from build123d import *

# Parameters (mm, degrees)
CUBE006_W                    = 20
CUBE006_H                    = 10
CUBE006_DEPTH                = 20
CUBE006_ROLL_ANGLE           = 35
CUBE006_PLACEMENT_ANGLE      = -45
CUBE008_W                    = 20
CUBE008_H                    = 10
CUBE008_DEPTH                = 20
CUBE008_ROLL_ANGLE           = 35
CUBE008_PLACEMENT_ANGLE      = -45
CUBE007_W                    = 20
CUBE007_H                    = 10
CUBE007_DEPTH                = 20
CUBE007_ROLL_ANGLE           = 35
CUBE007_PLACEMENT_ANGLE      = 45
CUBE005_W                    = 20
CUBE005_H                    = 10
CUBE005_DEPTH                = 20
CUBE005_ROLL_ANGLE           = 35
CUBE005_PLACEMENT_ANGLE      = 45
CUBE003_W                    = 4.5
CUBE003_H                    = 20
CUBE003_DEPTH                = 1.5
CUBE004_W                    = 4.5
CUBE004_H                    = 20
CUBE004_DEPTH                = 1.5
CYLINDER005_R                = 12
CYLINDER005_DEPTH            = 5
CYLINDER004_R                = 15
CYLINDER004_DEPTH            = 3.9
CUBE002_W                    = 4
CUBE002_H                    = 20
CUBE002_DEPTH                = 28.5
CYLINDER003_R                = 7.9
CYLINDER003_DEPTH            = 32.5
CUBE001_W                    = 10
CUBE001_H                    = 20
CUBE001_DEPTH                = 28.5
MATRIX_UNION_PITCH_ANGLE     = -90
MATRIX_UNION_PLACEMENT_ANGLE = 90
PRISM003_DEPTH               = 10
CYLINDER001_R                = 12
CYLINDER001_DEPTH            = 5
CYLINDER_R                   = 15
CYLINDER_DEPTH               = 3.9
DIFFERENCE_PITCH_ANGLE       = -90
DIFFERENCE_PLACEMENT_ANGLE   = 90
PRISM002_DEPTH               = 10
PRISM_DEPTH                  = 3
PRISM_PLACEMENT_ANGLE        = 30
PRISM001_DEPTH               = 3
PRISM001_PLACEMENT_ANGLE     = 30
CUBE_W                       = 26
CUBE_H                       = 14
CUBE_DEPTH                   = 3


with BuildPart() as cube006:
    # cube006 → cube006 (new body)
    with BuildSketch(Plane.XY):
        with Locations((10, 5)):
            Rectangle(CUBE006_W, CUBE006_H)
    extrude(amount=CUBE006_DEPTH)


with BuildPart() as cube006_1:
    # cube006 roll: moved
    add(cube006.part.rotate(Axis((0, 0, 0), (1, 0, 0)), CUBE006_ROLL_ANGLE))


with BuildPart() as cube006_2:
    # cube006 placement: moved
    add(cube006_1.part.moved(Location((-15.80755, -5.915414, -13.927285))).rotate(Axis((-15.80755, -5.915414, -13.927285), (0, 0, 1)), CUBE006_PLACEMENT_ANGLE))


with BuildPart() as cube008:
    # cube008 → cube008 (new body)
    with BuildSketch(Plane.XY):
        with Locations((10, 5)):
            Rectangle(CUBE008_W, CUBE008_H)
    extrude(amount=CUBE008_DEPTH)


with BuildPart() as cube008_1:
    # cube008 roll: moved
    add(cube008.part.rotate(Axis((0, 0, 0), (1, 0, 0)), CUBE008_ROLL_ANGLE))


with BuildPart() as cube008_2:
    # cube008 placement: moved
    add(cube008_1.part.moved(Location((-15.80755, -5.915414, -13.927285))).rotate(Axis((-15.80755, -5.915414, -13.927285), (0, 0, 1)), CUBE008_PLACEMENT_ANGLE))


with BuildPart() as matrix_union001:
    # cube007 → cube007 (new body)
    with BuildSketch(Plane.XY):
        with Locations((10, 5)):
            Rectangle(CUBE007_W, CUBE007_H)
    extrude(amount=CUBE007_DEPTH)


with BuildPart() as matrix_union001_1:
    # cube007 roll: moved
    add(matrix_union001.part.rotate(Axis((0, 0, 0), (1, 0, 0)), CUBE007_ROLL_ANGLE))


with BuildPart() as matrix_union001_2:
    # cube007 placement: moved
    add(matrix_union001_1.part.moved(Location((1.665414, -20.05755, -13.927285))).rotate(Axis((1.665414, -20.05755, -13.927285), (0, 0, 1)), CUBE007_PLACEMENT_ANGLE))

    # Matrix_Union001: union cube008
    add(cube008_2.part)


with BuildPart() as mirrored_matrix_union001:
    # mirr_Matrix_Union001: instance of Matrix_Union001
    add(matrix_union001_2.part.mirror(Plane(origin=(0, 0, 0), x_dir=(1, 0, 0), z_dir=(0, 1, 0))))


with BuildPart() as union005:
    # cube005 → cube005 (new body)
    with BuildSketch(Plane.XY):
        with Locations((10, 5)):
            Rectangle(CUBE005_W, CUBE005_H)
    extrude(amount=CUBE005_DEPTH)


with BuildPart() as union005_1:
    # cube005 roll: moved
    add(union005.part.rotate(Axis((0, 0, 0), (1, 0, 0)), CUBE005_ROLL_ANGLE))


with BuildPart() as union005_2:
    # cube005 placement: moved
    add(union005_1.part.moved(Location((1.665414, -20.05755, -13.927285))).rotate(Axis((1.665414, -20.05755, -13.927285), (0, 0, 1)), CUBE005_PLACEMENT_ANGLE))

    # union005: union cube006, mirrored Matrix_Union001
    add(cube006_2.part)
    add(mirrored_matrix_union001.part)


with BuildPart() as cube003:
    # cube003 → cube003 (new body)
    with BuildSketch(Plane(origin=(-10, -10, 0), x_dir=(1, 0, 0), z_dir=(0, 0, 1))):
        with Locations((2.25, 10)):
            Rectangle(CUBE003_W, CUBE003_H)
    extrude(amount=CUBE003_DEPTH)


with BuildPart() as cube004:
    # cube004 → cube004 (new body)
    with BuildSketch(Plane(origin=(-10, -10, 27), x_dir=(1, 0, 0), z_dir=(0, 0, 1))):
        with Locations((2.25, 10)):
            Rectangle(CUBE004_W, CUBE004_H)
    extrude(amount=CUBE004_DEPTH)


with BuildPart() as cylinder006:
    # cylinder006 → cylinder006 (revolve)
    with BuildSketch(Plane(origin=(0, 0, 3), x_dir=(1, 0, 0), z_dir=(0, -1, 0))):
        Polygon((0, 0), (12, 0), (15, 1), (0, 1), align=None)
    revolve(axis=Axis((0, 0, 3), (0, 0, 1)))


with BuildPart() as union004:
    # cylinder005 → cylinder005 (new body)
    with BuildSketch(Plane.XY):
        Circle(CYLINDER005_R)
    extrude(amount=CYLINDER005_DEPTH)

    # union004: union cylinder006
    add(cylinder006.part)


with BuildPart() as difference003:
    # cylinder004 → cylinder004 (new body)
    with BuildSketch(Plane.XY):
        Circle(CYLINDER004_R)
    extrude(amount=CYLINDER004_DEPTH)

    # difference003: cut union004
    add(union004.part, mode=Mode.SUBTRACT)


with BuildPart() as difference003_1:
    # difference003 placement: moved
    add(difference003.part.moved(Location((0, 0, 12.5))))


with BuildPart() as cube002:
    # cube002 → cube002 (new body)
    with BuildSketch(Plane(origin=(-14, -10, 0), x_dir=(1, 0, 0), z_dir=(0, 0, 1))):
        with Locations((2, 10)):
            Rectangle(CUBE002_W, CUBE002_H)
    extrude(amount=CUBE002_DEPTH)


with BuildPart() as cylinder003:
    # cylinder003 → cylinder003 (new body)
    with BuildSketch(Plane.XY.offset(-2)):
        Circle(CYLINDER003_R)
    extrude(amount=CYLINDER003_DEPTH)


with BuildPart() as difference005:
    # cube001 → cube001 (new body)
    with BuildSketch(Plane(origin=(-10, -10, 0), x_dir=(1, 0, 0), z_dir=(0, 0, 1))):
        with Locations((5, 10)):
            Rectangle(CUBE001_W, CUBE001_H)
    extrude(amount=CUBE001_DEPTH)

    # difference002: cut cylinder003
    add(cylinder003.part, mode=Mode.SUBTRACT)

    # union003: union cube002
    add(cube002.part)

    # difference004: cut difference003
    add(difference003_1.part, mode=Mode.SUBTRACT)

    # Matrix_Union: union cube003, cube004
    add(cube003.part)
    add(cube004.part)


with BuildPart() as difference005_1:
    # Matrix_Union pitch: moved
    add(difference005.part.rotate(Axis((0, 0, 0), (0, 1, 0)), MATRIX_UNION_PITCH_ANGLE))


with BuildPart() as difference005_2:
    # Matrix_Union placement: moved
    add(difference005_1.part.moved(Location((0, 14.25, 14))).rotate(Axis((0, 14.25, 14), (0, 0, 1)), MATRIX_UNION_PLACEMENT_ANGLE))

    # difference005: cut union005
    add(union005_2.part, mode=Mode.SUBTRACT)


with BuildPart() as prism003:
    # prism003 → prism003 (new body)
    with BuildSketch(Plane(origin=(14, 0, -0.1), x_dir=(1, 0, 0), z_dir=(0, 0, 1))):
        Polygon((1.7, 0), (1.570595, 0.650562), (1.202082, 1.202082), (0.650562, 1.570595), (0, 1.7), (-0.650562, 1.570595), (-1.202082, 1.202082), (-1.570595, 0.650562), (-1.7, 0), (-1.570595, -0.650562), (-1.202082, -1.202082), (-0.650562, -1.570595), (0, -1.7), (0.650562, -1.570595), (1.202082, -1.202082), (1.570595, -0.650562), align=None)
    extrude(amount=PRISM003_DEPTH)


with BuildPart() as cylinder002:
    # cylinder002 → cylinder002 (revolve)
    with BuildSketch(Plane(origin=(0, 0, 3), x_dir=(1, 0, 0), z_dir=(0, -1, 0))):
        Polygon((0, 0), (12, 0), (15, 1), (0, 1), align=None)
    revolve(axis=Axis((0, 0, 3), (0, 0, 1)))


with BuildPart() as union001:
    # cylinder001 → cylinder001 (new body)
    with BuildSketch(Plane.XY):
        Circle(CYLINDER001_R)
    extrude(amount=CYLINDER001_DEPTH)

    # union001: union cylinder002
    add(cylinder002.part)


with BuildPart() as difference:
    # cylinder → cylinder (new body)
    with BuildSketch(Plane.XY):
        Circle(CYLINDER_R)
    extrude(amount=CYLINDER_DEPTH)

    # difference: cut union001
    add(union001.part, mode=Mode.SUBTRACT)


with BuildPart() as difference_1:
    # difference pitch: moved
    add(difference.part.rotate(Axis((0, 0, 0), (0, 1, 0)), DIFFERENCE_PITCH_ANGLE))


with BuildPart() as difference_2:
    # difference placement: moved
    add(difference_1.part.moved(Location((0, 1.75, 14))).rotate(Axis((0, 1.75, 14), (0, 0, 1)), DIFFERENCE_PLACEMENT_ANGLE))


with BuildPart() as union002:
    # prism002 → prism002 (new body)
    with BuildSketch(Plane(origin=(-14, 0, -0.1), x_dir=(1, 0, 0), z_dir=(0, 0, 1))):
        Polygon((1.7, 0), (1.570595, 0.650562), (1.202082, 1.202082), (0.650562, 1.570595), (0, 1.7), (-0.650562, 1.570595), (-1.202082, 1.202082), (-1.570595, 0.650562), (-1.7, 0), (-1.570595, -0.650562), (-1.202082, -1.202082), (-0.650562, -1.570595), (0, -1.7), (0.650562, -1.570595), (1.202082, -1.202082), (1.570595, -0.650562), align=None)
    extrude(amount=PRISM002_DEPTH)

    # union002: union prism003, difference
    add(prism003.part)
    add(difference_2.part)


with BuildPart() as prism:
    # prism → prism (new body)
    with BuildSketch(Plane.XY):
        Polygon((7, 0), (3.5, 6.062178), (-3.5, 6.062178), (-7, 0), (-3.5, -6.062178), (3.5, -6.062178), align=None)
    extrude(amount=PRISM_DEPTH)


with BuildPart() as prism_1:
    # prism placement: moved
    add(prism.part.moved(Location((-13, 0, 0))).rotate(Axis((-13, 0, 0), (0, 0, 1)), PRISM_PLACEMENT_ANGLE))


with BuildPart() as prism001:
    # prism001 → prism001 (new body)
    with BuildSketch(Plane.XY):
        Polygon((7, 0), (3.5, 6.062178), (-3.5, 6.062178), (-7, 0), (-3.5, -6.062178), (3.5, -6.062178), align=None)
    extrude(amount=PRISM001_DEPTH)


with BuildPart() as prism001_1:
    # prism001 placement: moved
    add(prism001.part.moved(Location((13, 0, 0))).rotate(Axis((13, 0, 0), (0, 0, 1)), PRISM001_PLACEMENT_ANGLE))


with BuildPart() as group:
    # cube → cube (new body)
    with BuildSketch(Plane(origin=(-13, -7, 0), x_dir=(1, 0, 0), z_dir=(0, 0, 1))):
        with Locations((13, 7)):
            Rectangle(CUBE_W, CUBE_H)
    extrude(amount=CUBE_DEPTH)

    # union: union prism, prism001
    add(prism_1.part)
    add(prism001_1.part)

    # difference001: cut union002
    add(union002.part, mode=Mode.SUBTRACT)

    # Group: union difference005
    add(difference005_2.part)


solid = group.part
Input: part model. Units: mm. Frame: model coordinates. A direction names the side the tool comes from. Coordinates: 2 decimals unless noted, no trailing zeros. Loops run counter-clockwise (first coordinate to the right, second up) from the corner with the lowest first, then second, coordinate; pieces in that order, holes last.
(1) Section A-A on z = 11. Return the cut outline in (x, y).
(2) Pull-direction query (X, two-part tool) for faces 4 (the face through (-8.19, -12.35, 2.31)), 5 (the face through (11, 7, 1)), 6 (the face through (-0.17, 0.2, 6.1)), 7 (the face through (0, 12.75, 8)); classes: released by +X, released by -X, zero draft, split by the parting line, or undercut.
(3) Section D-D on z = 1. Count the separate pieces of the cut face and the enclosed holes in it, then the cut area to 3 significant figures.
(4) Material intervals for probe 1 along X at (y, z) = (9, 7.5); probe 2 along Y at (x, z) = (8, 5); probe 3 along X at (y, z) = (-0.5, 4.25), sorted ascending.
(5) First-contact query: pin 1 Ø2.5 at (x, z) = (-11, 2) entering from +Y; pin 2 Ø1 at (y, z) = (0, 9.5) entering from -X; pin 3 Ø1.5 at (x, z) = (11.5, 2) entering from +Y. Flat tips, straight axial feed; report the tip coordinate or a pass-through.
(6) Section B-B on x = 0. Return the cut outline in (y, z).
(7) Set-up query: faces 1 (the face through (-0.168, -1.306, 1.832)), 2 (the face through (15.989, -5.275, 1.479)), 3 (the face through (0, -12.75, 8)). Return all of +Z, -Z, +X, -X, +Y, -Y with unobstructed straight access to the full face (end or side cutting, diameter ignored); none if empty.
(8) Section C-C on y = -4.5. Return the cut outline in (x, z).
Data:
1. outline: (-10, -14.25) - (-7.31, -14.25) - (-7.31, 14.25) - (-10, 14.25) - close; (7.31, -14.25) - (10, -14.25) - (10, 14.25) - (7.31, 14.25) - close
2. face 4: released by -X
2. face 5: zero draft
2. face 6: undercut
2. face 7: undercut
3. separate pieces: 1
3. enclosed holes: 3
3. area: 660 mm2
4. probe 1: x = -10 to -4.49, 4.49 to 10
4. probe 2: y = -14.25 to -1.26, 1.75 to 14.25
4. probe 3: x = -7 to 7
5. pin 1: stops at y = 10.97
5. pin 2: stops at x = -10
5. pin 3: stops at y = 7
6. outline: (-14.25, 0) - (-1.92, 0) - (-1.25, 2) - (1.75, 2) - (1.75, 0) - (14.25, 0) - (14.25, 8.5) - (12.75, 8.5) - (12.75, 6.1) - (-12.75, 6.1) - (-12.75, 8.5) - (-14.25, 8.5) - close
7. face 1: none
7. face 2: +Z, -Z, +X, -Y
7. face 3: +Z
8. outline: (-17.33, 0) - (17.33, 0) - (17.33, 3) - (10, 3) - (10, 14) - (7.9, 14) arc R7.9 cw to (-7.9, 14) - (-10, 14) - (-10, 3) - (-17.33, 3) - close
